Part model, mm, in its own coordinate system. Coordinates: 2 decimals unless noted, no trailing zeros. Write each loop counter-clockwise with the first axis right and the second up, starting at its lowest first coordinate (ties: lowest second). Pieces come first, ordered by that corner, then holes. Notation, with made-up numbers: (5, 15.25) -> (51, 15.25) arc R26 ccw to (51, 41.25) -> close; hole circle Ø10 at (80.25, 57). An arc over 180 degrees is marked (long way). Write item = value, one per line. Start each with the question number.
Q1. Pin check, flat tips, straight feed: P1, Ø0.8, axis at y = -76.5, z = 0.5, coming from the +X side; P2, Ø0.8, axis at y = -1, z = 1, coming from the -X side. Stop position of each tip, or through.
Q2. Band-saw the part on C-C, the plane x = 223.5. List the corners of the cut face in (y, z).
Q3. Band-saw the part on D-D, the plane y = -27. List the corners of the cut face in (x, z), plus the area to 3 significant figures.
Q4. Probe line 1 (Y direction, x = 265, z = 1.15); line 2 (Y direction, x = 240.5, z = 1.1); line 3 (Y direction, x = 224, z = 0.45). List the from-to ranges inside material, lowest first.
Q5. Band-saw the part on A-A, the plane x = 263. List the corners of the cut face in (y, z).
Q6. Band-saw the part on B-B, the plane x = 241. List the corners of the cut face in (y, z), plus the area to 3 significant figures.
from build123d import *

# Parameters (mm, degrees)
BOSS_EXTRUDE1_DEPTH = 1.524


with BuildPart() as part:
    # Sketch1 → Boss-Extrude1 (new body)
    with BuildSketch(Plane.XY):
        with BuildLine():
            Line((211.523731391, 0), (211.523731391, -2.54))
            Line((211.523731391, -2.54), (202.922883793, -2.527561419))
            ThreePointArc((202.922883793, -2.527561419), (213.554085688, -12.168076331), (227.746163725, -14.300423044))
            ThreePointArc((227.746163725, -14.300423044), (229.650139274, -14.615955212), (231.019640286, -15.975789914))
            ThreePointArc((231.019640286, -15.975789914), (242.141029149, -26.800870517), (257.521078021, -28.879754104))
            ThreePointArc((257.521078021, -28.879754104), (259.093725099, -48.084230478), (275.202983438, -58.65669128))
            ThreePointArc((275.202983438, -58.65669128), (273.284119594, -63.70823493), (273.645185128, -69.099873213))
            ThreePointArc((273.645185128, -69.099873213), (273.142027669, -72.218330377), (270.098113996, -73.062446524))
            ThreePointArc((270.098113996, -73.062446524), (252.314484646, -72.190801616), (235.189633712, -67.316715223))
            ThreePointArc((235.189633712, -67.316715223), (231.709711317, -67.641087637), (229.865155612, -70.609705427))
            ThreePointArc((229.865155612, -70.609705427), (223.057551669, -74.973109583), (219.801437593, -82.374493805))
            ThreePointArc((219.801437593, -82.374493805), (235.189633712, -79.270242267), (250.709830302, -81.627455706))
            ThreePointArc((250.709830302, -81.627455706), (256.183079158, -82.374432464), (261.7070657, -82.374493805))
            ThreePointArc((261.7070657, -82.374493805), (273.347233029, -81.313035156), (284.987400357, -82.374493805))
            ThreePointArc((284.987400357, -82.374493805), (287.719421671, -80.411720704), (285.255147496, -78.121792432))
            ThreePointArc((285.255147496, -78.121792432), (284.981385526, -77.460846026), (284.73300841, -76.789947691))
            Line((284.73300841, -76.789947691), (254.383327933, -76.789947691))
            Line((254.383327933, -76.789947691), (254.383327933, -75.265947691))
            Line((254.383327933, -75.265947691), (284.273085104, -75.265947691))
            ThreePointArc((284.273085104, -75.265947691), (283.749737466, -69.068999992), (285.279905713, -63.041177943))
            Line((285.279905713, -63.041177943), (265.119779794, -35.456547246))
            Line((265.119779794, -35.456547246), (266.350198676, -34.557300131))
            Line((266.350198676, -34.557300131), (286.043441867, -61.503106065))
            ThreePointArc((286.043441867, -61.503106065), (286.989404718, -59.975403718), (288.077109535, -58.54515255))
            ThreePointArc((288.077109535, -58.54515255), (288.80590673, -53.43695911), (285.643381228, -49.359801029))
            ThreePointArc((285.643381228, -49.359801029), (274.368164292, -38.807208416), (272.826055023, -23.441349285))
            ThreePointArc((272.826055023, -23.441349285), (272.839039076, -21.86438539), (272.091685647, -20.475700197))
            ThreePointArc((272.091685647, -20.475700197), (270.245388722, -18.354306042), (268.523028934, -16.131109637))
            ThreePointArc((268.523028934, -16.131109637), (268.090816368, -15.671862862), (267.558783349, -15.333253695))
            ThreePointArc((267.558783349, -15.333253695), (264.150445583, -14.041396316), (260.57978956, -13.309223264))
            ThreePointArc((260.57978956, -13.309223264), (256.794003466, -10.41140001), (256.203064232, -5.680612889))
            ThreePointArc((256.203064232, -5.680612889), (256.293258056, -4.865684219), (256.119145106, -4.06447991))
            ThreePointArc((256.119145106, -4.06447991), (241.521161242, 12.295961664), (219.801437593, 15.299091023))
            Line((219.801437593, 15.299091023), (203.553625304, 8.095778667))
            Line((203.553625304, 8.095778667), (202.1481549, 0.013558997))
            Line((202.1481549, 0.013558997), (211.523731391, 0))
        make_face()
    extrude(amount=BOSS_EXTRUDE1_DEPTH)


solid = part.part
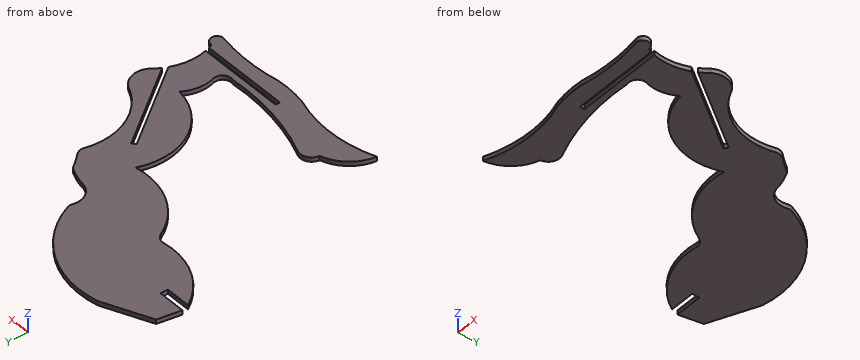
Ans:
q1.P1 = 284.77
q1.P2 = 211.52
q2.outline = (-81.11, 0) -> (-74.48, 0) -> (-74.48, 1.52) -> (-81.11, 1.52) -> close; (-14.55, 0) -> (15.88, 0) -> (15.88, 1.52) -> (-14.55, 1.52) -> close
q3.outline = (242.56, 0) -> (272.19, 0) -> (272.19, 1.52) -> (242.56, 1.52) -> close
q3.area = 45.2 mm2
q4.line_1 = -81.86 to -76.79, -75.27 to -73.23, -54.59 to -14.31
q4.line_2 = -79.45 to -69.29, -25.92 to 12.82
q4.line_3 = -80.96 to -73.97, -14.56 to 15.93
q5.outline = (-82.15, 0) -> (-76.79, 0) -> (-76.79, 1.52) -> (-82.15, 1.52) -> close; (-75.27, 0) -> (-73.2, 0) -> (-73.2, 1.52) -> (-75.27, 1.52) -> close; (-52.93, 0) -> (-13.74, 0) -> (-13.74, 1.52) -> (-52.93, 1.52) -> close
q6.outline = (-79.5, 0) -> (-69.45, 0) -> (-69.45, 1.52) -> (-79.5, 1.52) -> close; (-26.21, 0) -> (12.57, 0) -> (12.57, 1.52) -> (-26.21, 1.52) -> close
q6.area = 74.4 mm2
